Input: part model. Units: mm. Frame: model coordinates. Face numbers are marked on the shaded views. A direction names the side the tool comes from. Coordinates: 2 decimals unless noted, no trailing zeros. Loops run counter-clockwise (first coordinate to the right, second up) from the corner with the lowest first, then second, coordinate; pieces in that order, holes last. Notation, with made-up numbers: (-21.75, 49) - (-17.75, 49) arc R12 ccw to (-17.75, 62) - close; hole circle Ø4 at (63, 89.25). An arc over 180 degrees is marked (long way). Use one line per item in the form item = value.
from build123d import *

# Parameters (mm, degrees)
SKETCH5_W               = 0.5
SKETCH5_H               = 29
SKETCH5_H_2             = 27
BOSS_EXTRUDE1_DEPTH     = 0.25
SKETCH6_W               = 3.089069264
SKETCH6_H               = 11.690007215
CUT_EXTRUDE1_DEPTH      = 2.5
CUT_EXTRUDE2_DEPTH      = 30.534698967
CUT_EXTRUDE2_DEPTH_BACK = 30.534698967
SKETCH7_W               = 17.118012924
SKETCH7_H               = 27.873578567


with BuildPart() as part:
    # Sketch4 → Revolve1 (revolve)
    with BuildSketch(Plane(origin=(0, 0, 0), x_dir=(1, 0, 0), z_dir=(0, 1, 0))):
        with BuildLine():
            Line((-2.5, 4.771615798), (-2.5, -0.228384202))
            Line((-2.5, -0.228384202), (-3, -0.228384202))
            Line((-3, -0.228384202), (-3, -1.228384202))
            Line((-3, -1.228384202), (0, -1.228384202))
            Line((0, -1.228384202), (0, 7.271615798))
            ThreePointArc((0, 7.271615798), (-1.767766953, 6.539382751), (-2.5, 4.771615798))
        make_face()
    revolve(axis=Axis((0, 0, -8.02238806), (0, 0, 1)))

    # Sketch5 → Boss-Extrude1 (add, symmetric)
    with BuildSketch(Plane(origin=(0, 0, 0), x_dir=(1, 0, 0), z_dir=(0, 1, 0))):
        with Locations((-1.25, -14.728384202)):
            Rectangle(SKETCH5_W, SKETCH5_H)
        with Locations((1.25, -13.728384202)):
            Rectangle(SKETCH5_W, SKETCH5_H_2)
    extrude(amount=BOSS_EXTRUDE1_DEPTH, both=True)

    # Sketch6 → Cut-Extrude1 (cut, symmetric)
    with BuildSketch(Plane(origin=(0, 0, 0), x_dir=(1, 0, 0), z_dir=(0, 1, 0))):
        with Locations((4.044534632, -0.802626626)):
            Rectangle(SKETCH6_W, SKETCH6_H)
    extrude(amount=CUT_EXTRUDE1_DEPTH, both=True, mode=Mode.SUBTRACT)

    # Sketch7 → Cut-Extrude2 (cut, two sides: drawn at the far end of the back side and taken through both)
    with BuildSketch(Plane(origin=(0, 0, 0), x_dir=(1, 0, 0), z_dir=(0, 1, 0)).offset(-CUT_EXTRUDE2_DEPTH_BACK)):
        with Locations((0.81040788, -18.439111074)):
            Rectangle(SKETCH7_W, SKETCH7_H)
    extrude(amount=CUT_EXTRUDE2_DEPTH + CUT_EXTRUDE2_DEPTH_BACK, mode=Mode.SUBTRACT)


solid = part.part
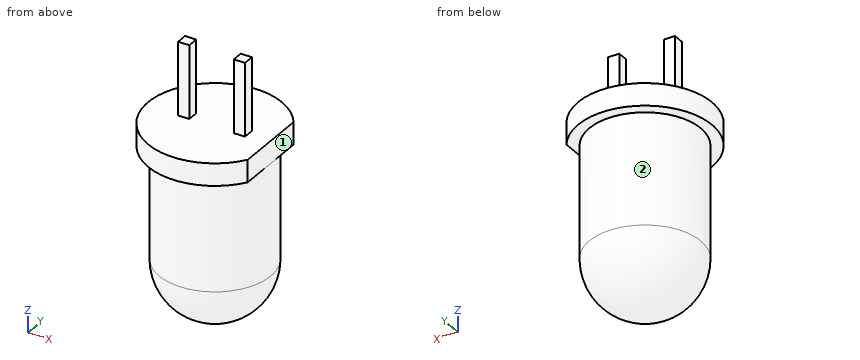
Q1. Cut plane A-A, the plane x = 0. Return loops of the section in (y, z).
Check values:
outline = (-3, 0.23) - (-2.5, 0.23) - (-2.5, -4.77) arc R2.5 ccw to (2.5, -4.77) - (2.5, 0.23) - (3, 0.23) - (3, 1.23) - (-3, 1.23) - close
Q2. Cut plane C-C, the plane z = -3.25. Return loops of the section in (x, y).
Check values:
outline = circle Ø5 at (0, 0)
Q3. Ray query, line 1 along Z through (x, y) = (-0.7, 2.7); line 2 along Y through (x, z) = (1.05, 1.75); line 3 along X through (y, z) = (-2, -2.5). Return the intervals inside material, ascending. Write a range as [from, to].
Check values:
line_1 = [0.23, 1.23]
line_2 = [-0.25, 0.25]
line_3 = [-1.5, 1.5]
Q4. Set-up query: the marked faces 1 and 2. Return all of +Z, -Z, +X, -X, +Y, -Y with unobstructed straight access to the full face (end or side cutting, diameter ignored); none if empty.
Check values:
face_1 = +Z, -Z, +X, +Y, -Y
face_2 = -Z
Q5. Cut plane B-B, the plane y = 0.5. Return loops of the section in (x, z), then the cut area to 3 significant figures.
Check values:
outline = (-2.96, 0.23) - (-2.45, 0.23) - (-2.45, -4.77) arc R2.45 ccw to (2.45, -4.77) - (2.45, 0.23) - (2.5, 0.23) - (2.5, 1.23) - (-2.96, 1.23) - close
area = 39.4 mm²
Q6. Cut plane D-D, the plane z = -6.5. Return loops of the section in (x, y).
Check values:
outline = circle Ø3.61 at (0, 0)
Q7. First-contact query: P1, Ø1.5, axis at x = -0.5, y = 1.5, coming from the +Z side; P2, Ø0.6, axis at x = -1.5, z = 3.5, coming from the +Y side; P3, Ø2, axis at x = 0.5, z = -1, coming from the -Y side. Flat tips, straight axial feed; report the tip coordinate or a pass-through.
Check values:
P1 = 1.23
P2 = 0.25
P3 = -2.5
